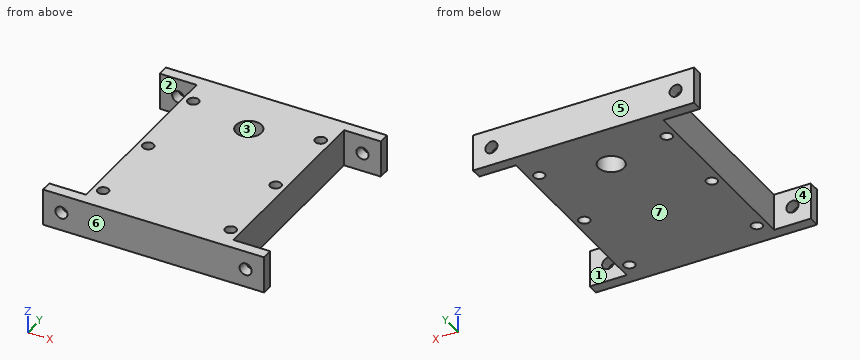
```python
from build123d import *

# Parameters (mm, degrees)
SKETCH1_W                    = 40
SKETCH1_H                    = 60
SKETCH1_R                    = 3.475
SKETCH1_R_2                  = 1.5
BOSS_EXTRUDE1_DEPTH          = 10
ESQUISSE1_W                  = 10
ESQUISSE1_H                  = 3
BOSS_EXTRU_1_DEPTH           = 10
ESQUISSE2_W                  = 10
ESQUISSE2_H                  = 3
BOSS_EXTRU_2_DEPTH           = 10
ENL_V_MAT_EXTRU_1_DEPTH      = 66.184353951
ENL_V_MAT_EXTRU_1_DEPTH_BACK = 66.184353951
ESQUISSE3_R                  = 1.65


with BuildPart() as part:
    # Sketch1 → Boss-Extrude1 (new body)
    with BuildSketch(Plane.XY):
        Rectangle(SKETCH1_W, SKETCH1_H)
        with Locations((0, 16.5)):
            Circle(SKETCH1_R, mode=Mode.SUBTRACT)
        with Locations((-17.3, -1.5)):
            Circle(SKETCH1_R_2, mode=Mode.SUBTRACT)
        with Locations((-17.3, 20.5)):
            Circle(SKETCH1_R_2, mode=Mode.SUBTRACT)
        with Locations(Location((17.3, -1.5, 0), (0, 0, 180))):
            Circle(SKETCH1_R_2, mode=Mode.SUBTRACT)
        with Locations(Location((17.3, 20.5, 0), (0, 0, 180))):
            Circle(SKETCH1_R_2, mode=Mode.SUBTRACT)
        with Locations((-17.3, -23.5)):
            Circle(SKETCH1_R_2, mode=Mode.SUBTRACT)
        with Locations(Location((17.3, -23.5, 0), (0, 0, 180))):
            Circle(SKETCH1_R_2, mode=Mode.SUBTRACT)
    extrude(amount=BOSS_EXTRUDE1_DEPTH)

    # Esquisse1 → Boss.-Extru.1 (add)
    with BuildSketch(Plane(origin=(20, 0, 0), x_dir=(0, 0, -1), z_dir=(1, 0, 0))):
        with Locations((-5, 28.5)):
            Rectangle(ESQUISSE1_W, ESQUISSE1_H)
        with Locations((-5, -28.5)):
            Rectangle(ESQUISSE1_W, ESQUISSE1_H)
    extrude(amount=BOSS_EXTRU_1_DEPTH)

    # Esquisse2 → Boss.-Extru.2 (add)
    with BuildSketch(Plane.ZY.offset(20)):
        with Locations((5, 28.5)):
            Rectangle(ESQUISSE2_W, ESQUISSE2_H)
        with Locations((5, -28.5)):
            Rectangle(ESQUISSE2_W, ESQUISSE2_H)
    extrude(amount=BOSS_EXTRU_2_DEPTH)

    # Esquisse3 → Enlèv. mat.-Extru.1 (cut, two sides: drawn at the far end of the back side and taken through both)
    with BuildSketch(Plane.XZ.offset(-27).offset(-ENL_V_MAT_EXTRU_1_DEPTH_BACK)):
        with Locations((-25, 5)):
            Circle(ESQUISSE3_R)
        with Locations((25, 5)):
            Circle(ESQUISSE3_R)
    extrude(amount=ENL_V_MAT_EXTRU_1_DEPTH + ENL_V_MAT_EXTRU_1_DEPTH_BACK, mode=Mode.SUBTRACT)


solid = part.part
```
Input: part model. Units: mm. Frame: model coordinates. Face numbers are marked on the shaded views. A direction names the side the tool comes from. Coordinates: 2 decimals unless noted, no trailing zeros. Write each loop counter-clockwise with the first axis right and the second up, starting at its lowest first coordinate (ties: lowest second). Pieces come first, ordered by that corner, then holes. Notation, with made-up numbers: (58, -30.75) -> (64, -30.75) arc R28 ccw to (64, -0.75) -> close; hole circle Ø7 at (-19.5, 40.25). An arc over 180 degrees is marked (long way). Answer as a JSON object with one key per item and string values.
1. First-contact query: P1, Ø5, axis at y = -6, z = 3.5, coming from the -X side; P2, Ø5, axis at x = -24, z = 4, coming from the +Y side; P3, Ø1.5, axis at y = 6, z = 9, coming from the +X side. Flat tips, straight axial feed; report the tip coordinate or a pass-through.
Result set:
{"P1": "stops at x = -20", "P2": "stops at y = 30", "P3": "stops at x = 20"}
2. Section C-C on y = -23.5. Return the cut outline in (x, z).
Result set:
{"outline": "(-20, 0) -> (-18.8, 0) -> (-18.8, 10) -> (-20, 10) -> close; (-15.8, 0) -> (15.8, 0) -> (15.8, 10) -> (-15.8, 10) -> close; (18.8, 0) -> (20, 0) -> (20, 10) -> (18.8, 10) -> close"}
3. Section A-A on y = 16.5. Return the cut outline in (x, z) (3 decimals), then the cut area to 4 significant figures.
Result set:
{"outline": "(-20, 0) -> (-3.475, 0) -> (-3.475, 10) -> (-20, 10) -> close; (3.475, 0) -> (20, 0) -> (20, 10) -> (3.475, 10) -> close", "area": "330.5 mm2"}
4. Section B-B on x = -25. Return the cut outline in (y, z).
Result set:
{"outline": "(-30, 0) -> (-27, 0) -> (-27, 3.35) -> (-30, 3.35) -> close; (-30, 6.65) -> (-27, 6.65) -> (-27, 10) -> (-30, 10) -> close; (27, 0) -> (30, 0) -> (30, 3.35) -> (27, 3.35) -> close; (27, 6.65) -> (30, 6.65) -> (30, 10) -> (27, 10) -> close"}
5. Section D-D on z = 8.5. Return the cut outline in (x, y) (3 decimals).
Result set:
{"outline": "(-30, -30) -> (30, -30) -> (30, -27) -> (20, -27) -> (20, 27) -> (30, 27) -> (30, 30) -> (-30, 30) -> (-30, 27) -> (-20, 27) -> (-20, -27) -> (-30, -27) -> close; hole circle Ø3 at (-17.3, -23.5); hole circle Ø3 at (-17.3, -1.5); hole circle Ø3 at (-17.3, 20.5); hole circle Ø6.95 at (0, 16.5); hole circle Ø3 at (17.3, -23.5); hole circle Ø3 at (17.3, -1.5); hole circle Ø3 at (17.3, 20.5)"}
6. Access query for the marked faces 1, 2 and 3. Directions: +Z, -Z, +X, -X, +Y, -Y. A direction counts if a zero-diameter tool reaches every point of the face in a straight line with its end or side. Return the directions, or none.
Result set:
{"face 1": "+Z, -Z, +X", "face 2": "+Z, -Z, -X", "face 3": "+Z, -Z"}
7. Mould query, pull axis Y, two halves, no side actions, for the marked faces 4, 5, 6 and 7. Classes: released by +Y, released by -Y, zero draft, split by the parting line, or undercut.
Result set:
{"face 4": "undercut", "face 5": "released by +Y", "face 6": "released by -Y", "face 7": "zero draft"}
8. Material intervals for line 1 (Y direction, x = -17.3, z = 2.75); line 2 (X direction, y = -28.2, z = 5); line 3 (Y direction, x = 27.5, z = 9.75), sorted ascending. Write a range as from..to.
Result set:
{"line 1": "y = -30..-25, -22..-3, 0..19, 22..30", "line 2": "x = -30..-26.65, -23.35..23.35, 26.65..30", "line 3": "y = -30..-27, 27..30"}
